Read the model definition and answer for the solid it produces. Units are mm, in the model's axes. A direction names the side the tool comes from. Coordinates: 2 decimals unless noted, no trailing zeros. Order: outer loops, then holes, each group sorted by start corner. A loop starts at its lowest first (then second) coordinate and runs counter-clockwise, first axis right, second up. Notation, with made-up numbers: M 59.25,36 L 65.25,36 A27 cw 65.25,52 Z; hole C -34,21.25 d5. An arc over 180 degrees is marked long. One line per question, with ' | ' between items. Start each with the question number.
1) Find section B-B, the plane y = 25. Write down the section's boundary in (x, z).
2) Find section C-C, the plane z = -4.75. Write down the section's boundary in (x, y).
3) The mould has two halves that part along Z. Classify faces 6 (the face through (1.141, 0.532, 8.797)), 7 (the face through (10, 39, 4)), 8 (the face through (1.141, -0.532, -8.797)): +Z half, -Z half, draft (parallel to the pull), parting line (faces both ways), or undercut.
4) Find section A-A, the plane x = 12.5. Count the separate pieces of the cut face and the enclosed holes in it, plus the area to 3 significant figures.
5) Given P1, Ø5.5, axis at y = -16, z = 1.5, coming from the +X side; P2, Ø0.9, axis at x = 3, y = -35, coming from the -Z side; P3, Ø0.8, axis at x = 10, y = -38.5, coming from the +Z side, each flat-ended and moving along its own axis, determine where each tip first touches the part or whether it passes through.
6) Consider probe 1 along Y at (x, z) = (2.75, 1.25); probe 2 along Z at (x, y) = (12.25, 22); probe 3 along Y at (x, z) = (8.75, 5.75). Determine where each line is inside the solid, lowest interval first.
7) A tool of negligible diameter and unlimited length cuts with its end or side. For faces 1 (the face through (6, 39, 0)), 2 (the face through (13.85, -23.295, 6.804)), 3 (the face through (7, -39, 0)), 4 (the face through (14, 0, -8)), 5 (the face through (3, -32.5, 2)), from which of +Z, -Z, +X, -X, +Y, -Y can it reach the whole face along a straight path? Write none if from no direction.
Autodesk Inventor part; units mm, degrees
ref_plane "YZ Plane" through (0, 0, 0) normal (1, 0, 0) x (0, 1, 0)
ref_plane "XZ Plane" through (0, 0, 0) normal (0, 1, 0) x (-1, 0, 0)
ref_plane "XY Plane" through (0, 0, 0) normal (0, 0, 1) x (1, 0, 0)
sketch "Skizze1" plane through (0, 0, 0) normal (1, 0, 0) x (0, 1, 0)
  line L0 (40, -10) -> (-40, -10)
  line L1 (-40, -10) -> (-40, 10)
  line L2 (-40, 10) -> (40, 10)
  line L3 (40, 10) -> (40, -10)
  line L4 (40, -10) -> (-40, 10) construction
  line L5 (-40, -10) -> (40, 10) construction
  point P0 (0, 0)
  dimension "d0" = 80
  dimension "d1" = 20
extrude "Extrusion1" add sketch "Skizze1" along normal blind 14
sketch "Skizze2" plane through (14, 0, 0) normal (1, 0, 0) x (0, 0, -1)
  line L0 (7.5, 37.5) -> (-7.5, 37.5)
  line L1 (-7.5, 37.5) -> (-7.5, -37.5)
  line L2 (-7.5, -37.5) -> (7.5, -37.5)
  line L3 (7.5, -37.5) -> (7.5, 37.5)
  line L4 (7.5, 37.5) -> (-7.5, -37.5) construction
  line L5 (-7.5, 37.5) -> (7.5, -37.5) construction
  line L6 (10, 40) -> (-10, 40)
  point P0 (0, 0)
  dimension "d4" = 15
  dimension "d5" = 2.5
extrude "Extrusion2" cut sketch "Skizze2" against normal blind 12
sketch "Skizze3" plane through (14, 0, 0) normal (1, 0, 0) x (0, 0, -1)
  line L0 (-2.7, -40) -> (2.5, -40)
  line L1 (2.5, -40) -> (2.5, -37.5)
  line L2 (2.5, -37.5) -> (-2.7, -37.5)
  line L3 (-2.7, -37.5) -> (-2.7, -40)
  line L4 (7.5, -37.5) -> (-7.5, -37.5)
  line L5 (-10, -40) -> (10, -40)
  line L6 (7.5, 37.5) -> (7.5, -37.5)
  point P0 (0, 0)
  dimension "d8" = 5.2
  dimension "d9" = 5
extrude "Extrusion3" cut sketch "Skizze3" against normal blind 7
sketch "Skizze4" plane through (2, 0, 0) normal (1, 0, 0) x (0, 0, -1)
  line L0 (5.5, -37.5) -> (7.5, -37.5)
  line L1 (7.5, -37.5) -> (7.5, -32.5)
  line L2 (7.5, -32.5) -> (5.5, -32.5)
  line L3 (5.5, -32.5) -> (5.5, -37.5)
  line L4 (7.5, -37.5) -> (-7.5, -37.5)
  line L5 (7.5, 37.5) -> (7.5, -37.5)
  line L6 (3.7, -37.5) -> (-7.5, -37.5)
  line L7 (-7.5, -37.5) -> (-7.5, -32.5)
  line L8 (-7.5, -32.5) -> (3.7, -32.5)
  line L9 (3.7, -32.5) -> (3.7, -37.5)
  line L10 (-7.5, -37.5) -> (-7.5, 37.5)
  line L11 (7.5, 14.5) -> (5.5, 14.5)
  line L12 (5.5, 14.5) -> (5.5, 19.5)
  line L13 (5.5, 19.5) -> (7.5, 19.5)
  line L14 (7.5, 19.5) -> (7.5, 14.5)
  line L15 (3.7, 14.5) -> (-7.5, 14.5)
  line L16 (-7.5, 14.5) -> (-7.5, 19.5)
  line L17 (-7.5, 19.5) -> (3.7, 19.5)
  line L18 (3.7, 19.5) -> (3.7, 14.5)
  line L19 (7.5, 19.5) -> (-7.5, 19.5)
  line L20 (-7.5, 19.5) -> (-7.5, 21.5)
  line L21 (-7.5, 21.5) -> (7.5, 21.5)
  line L22 (7.5, 21.5) -> (7.5, 19.5)
  point P0 (0, 0)
  dimension "d12" = 5
  dimension "d13" = 2
  dimension "d14" = 1.8
  dimension "d15" = 57
  dimension "d24" = 2
extrude "Extrusion4" add sketch "Skizze4" along normal blind 3 contours L3 L2 L1 L0 | L4 L7 L8 L9 | L11 L12 L13 L5 | L13 L19 L17 L10 L21 L5 | L10 L17 L18 L15
fillet "Rundung1" radius 2 4 edges at (2, -9, 7.5) (2, -9, -7.5) (2, 29.5, 7.5) (2, 29.5, -7.5)
fillet "Rundung2" radius 4 2 edges at (0, 0, 10) (0, 0, -10)
sketch "Skizze5" plane through (14, 0, 0) normal (1, 0, 0) x (0, 0, -1)
  line L0 (-4, 37.5) -> (4, 37.5)
  line L1 (4, 37.5) -> (4, 40)
  line L2 (4, 40) -> (-4, 40)
  line L3 (-4, 40) -> (-4, 37.5)
  line L4 (-7.5, 37.5) -> (7.5, 37.5)
  line L5 (10, 40) -> (-10, 40)
  line L6 (-6, 40) -> (6, 40)
  point P0 (0, 0)
  point P1 (0, 40)
  point P2 (0, 40)
  dimension "d20" = 8
extrude "Extrusion5" cut sketch "Skizze5" against normal blind 8
fillet "Rundung3" radius 2 10 edges at (0, 40, 0) (1.1716, 40, -8.8284) (9, 40, -10) (1.1716, 40, 8.8284) (9, 40, 10) (1.1716, -40, 8.8284) (9, -40, 10) (1.1716, -40, -8.8284) (9, -40, -10) (0, -40, 0)
sketch "Skizze6" plane through (14, 0, 0) normal (1, 0, 0) x (0, 0, -1)
  line L0 (-7.5, -37.5) -> (-7.5, 37.5)
  line L1 (-7.5, -26.7158) -> (-7.5, 11.7158)
  line L2 (-7.5, 11.7158) -> (-4.2, 6)
  line L3 (-7.5, -26.7158) -> (-4.2, -21)
  line L4 (-4.2, -21) -> (-4.2, 6)
  line L5 (-7.5, -7.5) -> (-4.2, -7.5) construction
  line L6 (-2.7, -40) -> (-2.7, -37.5) construction
  line L7 (-8, -40) -> (-2.7, -40) construction
  point P0 (0, 0)
  dimension "d25" = 27
  dimension "d26" = 30
  dimension "d27" = 1.5
  dimension "d28" = 19
extrude "Extrusion6" add sketch "Skizze6" against normal up to next
sketch "Skizze7" plane through (14, 0, 0) normal (1, 0, 0) x (0, 0, -1)
  line L0 (-4.2, 6) -> (-4.2, -21)
  line L1 (-4.2, -18.5) -> (-10, -28.5459)
  line L2 (-10, -38) -> (-10, 38)
  line L3 (-4.2, 3.5) -> (-10, 13.5459)
  line L4 (-10, 13.5459) -> (-10, -28.5459)
  line L5 (-4.2, 3.5) -> (-4.2, -18.5)
  line L6 (-10, -7.5) -> (-4.2, -7.5) construction
  line L7 (-4.2, -21) -> (-7.5, -26.7158)
  point P0 (0, 0)
  dimension "d31" = 22
extrude "Extrusion7" cut sketch "Skizze7" against normal blind 7.5
fillet "Rundung4" radius 2 1 edges at (6.5, -7.5, 10)
fillet "Rundung6" radius 2 4 edges at (5.5, -28.5459, 10) (10.25, -28.5459, 10) (5.5, 13.5459, 10) (10.25, 13.5459, 10)
fillet "Rundung5" radius 0.5 11 edges at (14, -39.4142, 9.4142) (14, -40, 5.35) (14, -33.5409, 10) (14, 39.4142, 9.4142) (14, 40, 6) (14, 26.0409, 10) (14, 39.4142, -9.4142) (14, 40, -6) (14, -39.4142, -9.4142) (14, -40, -5.25) (14, 0, -10)
equation "\"G_L\" = 0"
equation "\"G_H\" = 0"
equation "\"G_B\" = 0"
properties part number "5V_Supply" material "GEDA Stahl"
Report:
1) outline: M 0,-6 A4 ccw 4,-10 L 13.5,-10 A0.5 ccw 14,-9.5 L 14,-7.5 L 4,-7.5 A2 cw 2,-5.5 L 2,5.5 A2 cw 4,7.5 L 14,7.5 L 14,9.5 A0.5 ccw 13.5,10 L 4,10 A4 ccw 0,6 Z
2) outline: M 0,-38 A2 ccw 2,-40 L 13.5,-40 A0.5 ccw 14,-39.5 L 14,-37.5 L 2,-37.5 L 2,19.5 L 5,19.5 L 5,21.5 L 2,21.5 L 2,37.5 L 14,37.5 L 14,39.5 A0.5 ccw 13.5,40 L 2,40 A2 ccw 0,38 Z
3) face 6: +Z half | face 7: undercut | face 8: -Z half
4) separate pieces: 3 | enclosed holes: 0 | area: 361 mm^2
5) P1: stops at x = 6.5 | P2: stops at z = -9.96 | P3: stops at z = 10
6) probe 1: y = -40 to -32.5, 14.5 to 21.5, 37.5 to 40 | probe 2: z = -10 to -7.5, 7.5 to 10 | probe 3: y = -40 to -37.5, -23.68 to -21.18, 6.18 to 8.68, 37.5 to 40
7) face 1: +X, +Y | face 2: +Z, +X | face 3: +X, +Y, -Y | face 4: +Z, -Z, +X, +Y, -Y | face 5: +X
